For this review, take the finished solid that the model builds, in its own axes (mm). A direction names the side the tool comes from. Give positions to 0.01 mm unless a question says otherwise; leave off trailing zeros. Loops run counter-clockwise (first coordinate to the right, second up) from the corner with the lowest first, then second, coordinate; pieces in that order, holes last. Notation, with made-up numbers: (-15.5, 34.25) - (21.5, 34.25) arc R20 ccw to (21.5, 44.25) - close; hole circle Ø9 at (73, 42.5). An arc over 180 degrees is marked (long way). Put each result on its own line as item: value. Start each with the question number.
from build123d import *

# Parameters (mm, degrees)
SKETCH1_W               = 212.5
SKETCH1_H               = 339.725
BOSS_EXTRUDE1_DEPTH     = 6
SKETCH2_W               = 6.5
SKETCH2_H               = 20
BOSS_EXTRUDE2_DEPTH     = 24
SKETCH3_R               = 4
CUT_EXTRUDE1_DEPTH      = 19.5
CUT_EXTRUDE1_DEPTH_BACK = 195
FILLET2_R               = 5
SKETCH5_R               = 3.175
CUT_EXTRUDE2_DEPTH      = 7
CUT_EXTRUDE3_DEPTH      = 7


with BuildPart() as part:
    # Sketch1 → Boss-Extrude1 (new body)
    with BuildSketch(Plane.XY):
        with Locations((106.25, -169.8625)):
            Rectangle(SKETCH1_W, SKETCH1_H)
    extrude(amount=BOSS_EXTRUDE1_DEPTH)

    # Sketch2 → Boss-Extrude2 (add)
    with BuildSketch(Plane.XY.offset(6)):
        with Locations((21.75, -35.2425)):
            Rectangle(SKETCH2_W, SKETCH2_H)
        with Locations((50.75, -35.2425)):
            Rectangle(SKETCH2_W, SKETCH2_H)
        with Locations((190.75, -35.2425)):
            Rectangle(SKETCH2_W, SKETCH2_H)
        with Locations((161.75, -35.2425)):
            Rectangle(SKETCH2_W, SKETCH2_H)
        with Locations((133.75, -104.5325)):
            Rectangle(SKETCH2_W, SKETCH2_H)
        with Locations((165.25, -104.5325)):
            Rectangle(SKETCH2_W, SKETCH2_H)
        with Locations((165.25, -235.1925)):
            Rectangle(SKETCH2_W, SKETCH2_H)
        with Locations((21.75, -304.4825)):
            Rectangle(SKETCH2_W, SKETCH2_H)
        with Locations((50.75, -304.4825)):
            Rectangle(SKETCH2_W, SKETCH2_H)
        with Locations((190.75, -304.4825)):
            Rectangle(SKETCH2_W, SKETCH2_H)
        with Locations((161.75, -304.4825)):
            Rectangle(SKETCH2_W, SKETCH2_H)
        with Locations((133.75, -235.1925)):
            Rectangle(SKETCH2_W, SKETCH2_H)
    extrude(amount=BOSS_EXTRUDE2_DEPTH)

    # Sketch3 → Cut-Extrude1 (cut, two sides)
    with BuildSketch(Plane.ZY.offset(-18.5)) as cut_extrude1_sk:
        with Locations((18, -35.2425)):
            Circle(SKETCH3_R)
        with Locations((18, -235.1925)):
            Circle(SKETCH3_R)
        with Locations((18, -304.4825)):
            Circle(SKETCH3_R)
        with Locations((18, -104.5325)):
            Circle(SKETCH3_R)
        with BuildLine():
            Line((18, -25.2425), (18, -12.982943413))
            Line((18, -12.982943413), (51.949532367, -12.982943413))
            Line((51.949532367, -12.982943413), (51.949532367, -57.481006387))
            Line((51.949532367, -57.481006387), (18, -57.481006387))
            Line((18, -57.481006387), (18, -45.2425))
            ThreePointArc((18, -45.2425), (28, -35.2425), (18, -25.2425))
        make_face()
        with BuildLine():
            Line((52.442304634, -132.399123951), (18, -132.399123951))
            Line((18, -132.399123951), (18, -114.5325))
            ThreePointArc((18, -114.5325), (28, -104.5325), (18, -94.5325))
            Line((18, -94.5325), (18, -71.59149594))
            Line((18, -71.59149594), (52.442304634, -71.59149594))
            Line((52.442304634, -71.59149594), (52.442304634, -132.399123951))
        make_face()
        with BuildLine():
            Line((52.599532243, -270.375386727), (18, -270.375386727))
            Line((18, -270.375386727), (18, -245.1925))
            ThreePointArc((18, -245.1925), (28, -235.1925), (18, -225.1925))
            Line((18, -225.1925), (18, -207.306351849))
            Line((18, -207.306351849), (52.599532243, -207.306351849))
            Line((52.599532243, -207.306351849), (52.599532243, -270.375386727))
        make_face()
        with BuildLine():
            Line((52.621034016, -326.721115515), (18, -326.721115515))
            Line((18, -326.721115515), (18, -314.4825))
            ThreePointArc((18, -314.4825), (28, -304.4825), (18, -294.4825))
            Line((18, -294.4825), (18, -282.222834285))
            Line((18, -282.222834285), (52.621034016, -282.222834285))
            Line((52.621034016, -282.222834285), (52.621034016, -326.721115515))
        make_face()
    extrude(amount=CUT_EXTRUDE1_DEPTH, mode=Mode.SUBTRACT)
    extrude(cut_extrude1_sk.sketch, amount=-CUT_EXTRUDE1_DEPTH_BACK, mode=Mode.SUBTRACT)

    # Fillet2
    fillet2_edges = [part.edges().sort_by_distance(p)[0] for p in [
        (190.75, -45.2425, 6),
        (194, -35.2425, 6),
        (190.75, -25.2425, 6),
        (50.75, -45.2425, 6),
        (54, -35.2425, 6),
        (50.75, -25.2425, 6),
        (21.75, -25.2425, 6),
        (18.5, -35.2425, 6),
        (21.75, -45.2425, 6),
        (161.75, -25.2425, 6),
        (158.5, -35.2425, 6),
        (161.75, -45.2425, 6),
        (161.75, -294.4825, 6),
        (161.75, -314.4825, 6),
        (158.5, -304.4825, 6),
        (190.75, -314.4825, 6),
        (194, -304.4825, 6),
        (190.75, -294.4825, 6),
        (165.25, -245.1925, 6),
        (168.5, -235.1925, 6),
        (165.25, -225.1925, 6),
        (133.75, -225.1925, 6),
        (130.5, -235.1925, 6),
        (133.75, -245.1925, 6),
        (50.75, -314.4825, 6),
        (54, -304.4825, 6),
        (50.75, -294.4825, 6),
        (21.75, -294.4825, 6),
        (21.75, -314.4825, 6),
        (18.5, -304.4825, 6),
        (165.25, -114.5325, 6),
        (165.25, -94.5325, 6),
        (168.5, -104.5325, 6),
        (133.75, -94.5325, 6),
        (130.5, -104.5325, 6),
        (133.75, -114.5325, 6),
    ]]
    fillet(fillet2_edges, radius=FILLET2_R)

    # Sketch5 → Cut-Extrude2 (cut, through all)
    with BuildSketch(Plane.XY.offset(6)):
        with Locations((12.7, -12.7)):
            Circle(SKETCH5_R)
        with Locations((199.8, -12.7)):
            Circle(SKETCH5_R)
        with Locations((146.25, -35.2425)):
            Circle(SKETCH5_R)
        with Locations((176.25, -57.8625)):
            Circle(SKETCH5_R)
        with Locations((36.25, -57.8625)):
            Circle(SKETCH5_R)
        with Locations((191.25, -104.5325)):
            Circle(SKETCH5_R)
        with Locations((36.25, -169.8625)):
            Circle(SKETCH5_R)
        with Locations((191.25, -169.8625)):
            Circle(SKETCH5_R)
        with Locations((36.25, -281.8625)):
            Circle(SKETCH5_R)
        with Locations((66.25, -304.4825)):
            Circle(SKETCH5_R)
        with Locations((12.7, -327.025)):
            Circle(SKETCH5_R)
        with Locations((199.8, -327.025)):
            Circle(SKETCH5_R)
        with Locations((146.25, -304.4825)):
            Circle(SKETCH5_R)
    extrude(amount=-CUT_EXTRUDE2_DEPTH, mode=Mode.SUBTRACT)

    # Sketch9 → Cut-Extrude3 (cut, through all)
    with BuildSketch(Plane.XY.offset(6)):
        with BuildLine():
            Line((70, -271.3625), (110, -271.3625))
            ThreePointArc((110, -271.3625), (114.242640687, -269.605140687), (116, -265.3625))
            Line((116, -265.3625), (116, -74.3625))
            ThreePointArc((116, -74.3625), (114.242640687, -70.119859313), (110, -68.3625))
            Line((110, -68.3625), (70, -68.3625))
            ThreePointArc((70, -68.3625), (65.757359313, -70.119859313), (64, -74.3625))
            Line((64, -74.3625), (64, -265.3625))
            ThreePointArc((64, -265.3625), (65.757359313, -269.605140687), (70, -271.3625))
        make_face()
    extrude(amount=-CUT_EXTRUDE3_DEPTH, mode=Mode.SUBTRACT)


solid = part.part
1) Wall thickness on probe 1 along Y at (x, z) = (51.75, 18); probe 2 along Y at (x, z) = (199.8, 1.45) (3 decimals); probe 3 along Y at (x, z) = (36.25, 3.45) (1 decimal): over which ranges is each line inside the solid? List them lowest first.
2) Machinability: for faces 1 (the flat face through (22, -314.482, 14)), 2 (the flat face through (165, -245.192, 14)), 3 (the flat face through (162, -232, 14)), 4 (the flat face through (47.5, -301, 14)), which of the approach directions +Z, -Z, +X, -X, +Y, -Y give a long, thin tool a straight path to every point of the face, cutting with its end or side? Answer none if there is none.
3) Take a section at A-A on y = -213.5. State the section outline as (x, z) points.
4) Mouldability with a two-part tool opening along Z and no side actions: class faces 5 (the cylindrical face through (161.704, -300.517, 17.479)), 6 (the cylindrical face through (21.704, -31.277, 17.479)), 7 (the flat face through (162, -314.482, 14)), 8 (the cylindrical face through (21.704, -35.462, 27.998)) as released by +Z, released by -Z, zero draft, split by the parting line, or undercut.
5) Take a section at B-B on x = 78.5. State the section outline as (y, z) points (1 decimal), and give its area (3 significant figures).
6) Insertion check: P1, Ø13.5, axis at y = -236.5, z = 16.5, coming from the +X side; P2, Ø5, axis at x = 123.5, y = -183, coming from the +Z side; P3, Ø13, axis at y = -304.48, z = 18, coming from the -X side. Each pin has a flat end and moves straight along its axis. Give the tip position at first contact, or say it passes through.
Answers follow:
1. probe 1: -314.48 to -308.48, -300.48 to -294.48, -45.24 to -39.24, -31.24 to -25.24
1. probe 2: -339.725 to -330.2, -323.85 to -15.875, -9.525 to 0
1. probe 3: -339.7 to -285, -278.7 to -173, -166.7 to -61, -54.7 to 0
2. face 1: +Z, +X, -X, -Y
2. face 2: +Z, +X, -X
2. face 3: +Z
2. face 4: +Z, +Y, -Y
3. outline: (0, 0) - (64, 0) - (64, 6) - (0, 6) - close; (116, 0) - (212.5, 0) - (212.5, 6) - (116, 6) - close
4. face 5: undercut
4. face 6: undercut
4. face 7: zero draft
4. face 8: released by +Z
5. outline: (-339.7, 0) - (-271.4, 0) - (-271.4, 6) - (-339.7, 6) - close; (-68.4, 0) - (0, 0) - (0, 6) - (-68.4, 6) - close
5. area: 820 mm2
6. P1: x = 168.66
6. P2: z = 6
6. P3: x = 18.5
